from build123d import *

# Parameters (mm, degrees)
BOSS_EXTRUDE1_DEPTH = 18
CUT_EXTRUDE1_REACH  = 40.177
SKETCH2_R           = 4
FILLET2_RADIUS      = 9
FILLET2_LENGTH      = 3
FILLET3_RADIUS      = 9
FILLET3_LENGTH      = 3


with BuildPart() as part:
    # Sketch1 → Boss-Extrude1 (new body)
    with BuildSketch(Plane.XY):
        with BuildLine():
            Line((31, 0), (15, 0))
            ThreePointArc((15, 0), (13.682550737, 0.495231765), (13.017544199, 1.73567256))
            ThreePointArc((13.017544199, 1.73567256), (0, 13.13274595), (-13.017544199, 1.73567256))
            ThreePointArc((-13.017544199, 1.73567256), (-13.682550737, 0.495231765), (-15, 0))
            Line((-15, 0), (-31, 0))
            Line((-31, 0), (-31, 3))
            Line((-31, 3), (-17.429758337, 3))
            ThreePointArc((-17.429758337, 3), (-16.226217084, 3.402662073), (-15.507296248, 4.448511548))
            ThreePointArc((-15.507296248, 4.448511548), (0, 16.13274595), (15.507296248, 4.448511548))
            ThreePointArc((15.507296248, 4.448511548), (16.226217084, 3.402662073), (17.429758337, 3))
            Line((17.429758337, 3), (31, 3))
            Line((31, 3), (31, 0))
        make_face()
    extrude(amount=BOSS_EXTRUDE1_DEPTH)

    # Sketch2 → Cut-Extrude1 (cut, up to next)
    with BuildSketch(Plane(origin=(0, 3, 0), x_dir=(1, 0, 0), z_dir=(0, 1, 0)), mode=Mode.PRIVATE) as cut_extrude1_sk1:
        with Locations(Location((-23, -9, 0), (0, 0, 180))):
            Circle(SKETCH2_R)
    cut_extrude1_tool1 = extrude(cut_extrude1_sk1.sketch, amount=-CUT_EXTRUDE1_REACH, mode=Mode.PRIVATE) & part.part
    # Sketch2 → Cut-Extrude1 (cut, up to next)
    with BuildSketch(Plane(origin=(0, 3, 0), x_dir=(1, 0, 0), z_dir=(0, 1, 0)), mode=Mode.PRIVATE) as cut_extrude1_sk2:
        with Locations(Location((23, -9, 0), (0, 0, 180))):
            Circle(SKETCH2_R)
    cut_extrude1_tool2 = extrude(cut_extrude1_sk2.sketch, amount=-CUT_EXTRUDE1_REACH, mode=Mode.PRIVATE) & part.part
    add(cut_extrude1_tool1.solids().sort_by_distance((-23, 3, 9))[0], mode=Mode.SUBTRACT)
    add(cut_extrude1_tool2.solids().sort_by_distance((23, 3, 9))[0], mode=Mode.SUBTRACT)

    # Fillet2: full round fillet: the end face becomes a half cylinder, R = half its width
    fillet2_face = Plane((-31, 1.5, 9), x_dir=(0, -1, 0), z_dir=(-1, 0, 0))  # on the end face: x along it, z out of the body
    fillet2_slab = fillet2_face.offset(-FILLET2_RADIUS / 2) * Box(FILLET2_LENGTH, 2 * FILLET2_RADIUS, FILLET2_RADIUS, mode=Mode.PRIVATE)  # the body's end, R deep
    fillet2_round = Plane((-22, 1.5, 9), x_dir=(-1, 0, 0), z_dir=(0, -1, 0)) * Cylinder(FILLET2_RADIUS, FILLET2_LENGTH, mode=Mode.PRIVATE)  # its axis R under the face
    add(fillet2_slab - fillet2_round, mode=Mode.SUBTRACT)

    # Fillet3: full round fillet: the end face becomes a half cylinder, R = half its width
    fillet3_face = Plane((31, 1.5, 9), x_dir=(0, 1, 0), z_dir=(1, 0, 0))  # on the end face: x along it, z out of the body
    fillet3_slab = fillet3_face.offset(-FILLET3_RADIUS / 2) * Box(FILLET3_LENGTH, 2 * FILLET3_RADIUS, FILLET3_RADIUS, mode=Mode.PRIVATE)  # the body's end, R deep
    fillet3_round = Plane((22, 1.5, 9), x_dir=(1, 0, 0), z_dir=(0, 1, 0)) * Cylinder(FILLET3_RADIUS, FILLET3_LENGTH, mode=Mode.PRIVATE)  # its axis R under the face
    add(fillet3_slab - fillet3_round, mode=Mode.SUBTRACT)


solid = part.part
Could you check a few things on this model? Use its own coordinates, in mm. A direction names the side the tool comes from. Give positions to 0.01 mm unless a question says otherwise; leave off trailing zeros. Write each loop counter-clockwise with the first axis right and the second up, starting at its lowest first coordinate (ties: lowest second). Pieces come first, ordered by that corner, then holes. Notation, with made-up numbers: (47.5, -37) -> (90.5, -37) arc R21 cw to (90.5, -18) -> close; hole circle Ø10 at (-13.5, 11). An arc over 180 degrees is marked (long way). Write each question's results on one line, items separated by ' | '. Start each with the question number.
Q1. Suppose I cut it at C-C, the plane x = 23. List the corners of the cut face in (y, z) for me, and give its area (3 significant figures).
Q2. I need wall thicknesses on probe 1 along Y at (x, z) = (21, 5.5); probe 2 along X at (y, z) = (9.5, 2.5); probe 3 along Z at (x, y) = (-23, 0.9). Which ranges of each line are inside material? Lowest first, please.
Q3. I'm going to push flat-ended pins straight in: pin 1 Ø7 at (x, z) = (-25.5, 9.5) entering from +Y; pin 2 Ø3 at (x, z) = (-7, 8) entering from -Y. Where does each tip first touch, or does it pass through?
Q4. Suppose I cut it at A-A, the plane z = 9. List the corners of the cut face in (x, y) for me, and give its area (3 significant figures).
Q5. Suppose I cut it at D-D, the plane z = 2. List the corners of the cut face in (x, y) for me, and give its area (3 significant figures).
Q6. We'd pull the mould along X, two halves only. Please class faces 4 (the face through (-0.29, 16.13, 8.87)), 5 (the face through (13.7, 0.48, 8.87)), 6 (the face through (-27.3, 3, 8.9)): +X half, -X half, draft (parallel to the pull), parting line (faces both ways), or undercut.
Q7. Which directions (+Z, -Z, +X, -X, +Y, -Y) give clear straight access to the entire face, cutting with the end or side of a thin tool? Please do faces 1 (the face through (24.1, 3, 4.9)), 2 (the face through (-13.667, 0.509, 8.874)), 3 (the face through (26.2, 1.5, 6.6)).
Q8. Suppose I cut it at B-B, the plane y = 10. List the corners of the cut face in (x, z) for me.
Outcome:
1) outline: (0, 0.06) -> (3, 0.06) -> (3, 5) -> (0, 5) -> close; (0, 13) -> (3, 13) -> (3, 17.94) -> (0, 17.94) -> close | area: 29.7 mm2
2) probe 1: 0 to 3 | probe 2: -13.04 to -9.07, 9.07 to 13.04 | probe 3: 0.06 to 5, 13 to 17.94
3) pin 1: y = 3 | pin 2: y = 10.01
4) outline: (-31, 0) -> (-27, 0) -> (-27, 3) -> (-31, 3) -> close; (-19, 0) -> (-15, 0) arc R2 ccw to (-13.02, 1.74) arc R13.13 cw to (13.02, 1.74) arc R2 ccw to (15, 0) -> (19, 0) -> (19, 3) -> (17.43, 3) arc R2 cw to (15.51, 4.45) arc R16.13 ccw to (-15.51, 4.45) arc R2 cw to (-17.43, 3) -> (-19, 3) -> close; (27, 0) -> (31, 0) -> (31, 3) -> (27, 3) -> close | area: 179 mm2
5) outline: (-27.66, 0) -> (-15, 0) arc R2 ccw to (-13.02, 1.74) arc R13.13 cw to (13.02, 1.74) arc R2 ccw to (15, 0) -> (27.66, 0) -> (27.66, 3) -> (17.43, 3) arc R2 cw to (15.51, 4.45) arc R16.13 ccw to (-15.51, 4.45) arc R2 cw to (-17.43, 3) -> (-27.66, 3) -> close | area: 207 mm2
6) face 4: parting line | face 5: undercut | face 6: draft
7) face 1: +Z, -Z, +X, +Y | face 2: +Z, -Z, -Y | face 3: +Y, -Y
8) outline: (-12.66, 0) -> (-8.51, 0) -> (-8.51, 18) -> (-12.66, 18) -> close; (8.51, 0) -> (12.66, 0) -> (12.66, 18) -> (8.51, 18) -> close
